For this review, take the finished solid that the model builds, in its own axes (mm). Face numbers are marked on the shaded views. Round coordinates to 2 decimals unless told otherwise and drop trailing zeros. Write each loop counter-clockwise with the first axis right and the second up, starting at its lowest first coordinate (ties: lowest second). Pieces come first, ordered by that corner, then holes.
from build123d import *

# Parameters (mm, degrees)
SKETCH1_W           = 112
SKETCH1_H           = 50
SKETCH1_R           = 11.5
SKETCH1_W_2         = 25
SKETCH1_R_2         = 2
BOSS_EXTRUDE1_DEPTH = 10


with BuildPart() as part:
    # Sketch1 → Boss-Extrude1 (new body)
    # profile 1 of 3: a face of its own
    with BuildSketch(Plane(origin=(0, 0, 0), x_dir=(0, 0, -1), z_dir=(1, 0, 0))):
        Rectangle(SKETCH1_W, SKETCH1_H)
        Circle(SKETCH1_R, mode=Mode.SUBTRACT)
    # profile 2 of 3: a face of its own
    with BuildSketch(Plane(origin=(0, 0, 0), x_dir=(0, 0, -1), z_dir=(1, 0, 0))):
        with Locations((-68.5, 0)):
            Rectangle(SKETCH1_W_2, SKETCH1_H)
        with Locations((-68.5, -10)):
            Circle(SKETCH1_R_2, mode=Mode.SUBTRACT)
        with Locations((-68.5, 10)):
            Circle(SKETCH1_R_2, mode=Mode.SUBTRACT)
    # profile 3 of 3: a face of its own
    with BuildSketch(Plane(origin=(0, 0, 0), x_dir=(0, 0, -1), z_dir=(1, 0, 0))):
        with Locations((68.5, 0)):
            Rectangle(SKETCH1_W_2, SKETCH1_H)
        with Locations((68.5, -10)):
            Circle(SKETCH1_R_2, mode=Mode.SUBTRACT)
        with Locations((68.5, 10)):
            Circle(SKETCH1_R_2, mode=Mode.SUBTRACT)
    extrude(amount=BOSS_EXTRUDE1_DEPTH)


solid = part.part
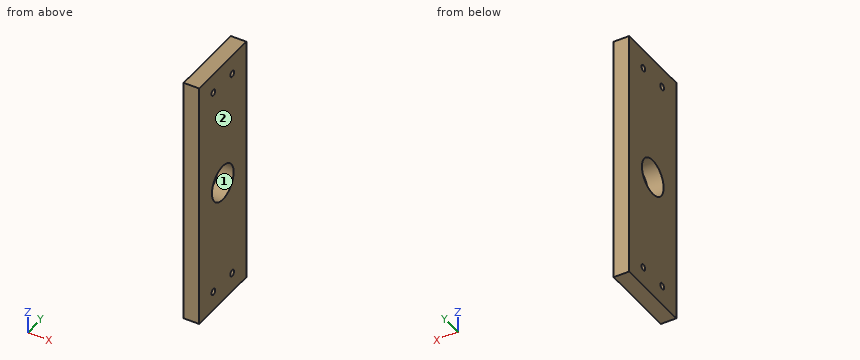
(1) For line 1 along Y through (x, z) = (7, -68.5); line 2 along Y through (x, z) = (6.25, -67); line 3 along Z through (x, y) = (9.5, 9), list the stretches that pass through material, from the lowest coordinate up.
Geometry check:
line 1: y = -25 to -12, -8 to 8, 12 to 25
line 2: y = -25 to -11.32, -8.68 to 8.68, 11.32 to 25
line 3: z = -81 to -70.23, -66.77 to -7.16, 7.16 to 66.77, 70.23 to 81
(2) We need section D-D, the plane z = 68.5. Give the boundary of the cut face in (x, y).
Geometry check:
outline: (0, -25) - (10, -25) - (10, -12) - (0, -12) - close; (0, -8) - (10, -8) - (10, 8) - (0, 8) - close; (0, 12) - (10, 12) - (10, 25) - (0, 25) - close
(3) Mouldability with a two-part tool opening along Y and no side actions: class the marked faces 1 and 2 as pulls with the +Y half, pulls with the -Y half, needs draft (parallel to the pull), parting line crosses it, or undercut.
Geometry check:
face 1: undercut
face 2: needs draft
(4) For pin 1 Ø2.5 at (y, z) = (10, 68.5) entering from +X, flat-tipped, find the tip position at first contact; note if it passes through.
Geometry check:
pin 1: passes through
(5) We need section B-B, the plane y = 0. Give the boundary of the cut face in (x, z), and give its area (3 significant figures).
Geometry check:
outline: (0, -81) - (10, -81) - (10, -11.5) - (0, -11.5) - close; (0, 11.5) - (10, 11.5) - (10, 81) - (0, 81) - close
area: 1,390 mm2
(6) We need section A-A, the plane z = 0. Give the boundary of the cut face in (x, y), and give its area (3 significant figures).
Geometry check:
outline: (0, -25) - (10, -25) - (10, -11.5) - (0, -11.5) - close; (0, 11.5) - (10, 11.5) - (10, 25) - (0, 25) - close
area: 270 mm2
(7) We need section C-C, the plane x = 5.5. Give the boundary of the cut face in (y, z).
Geometry check:
outline: (-25, -81) - (25, -81) - (25, 81) - (-25, 81) - close; hole circle Ø4 at (-10, -68.5); hole circle Ø4 at (-10, 68.5); hole circle Ø23 at (0, 0); hole circle Ø4 at (10, -68.5); hole circle Ø4 at (10, 68.5)
